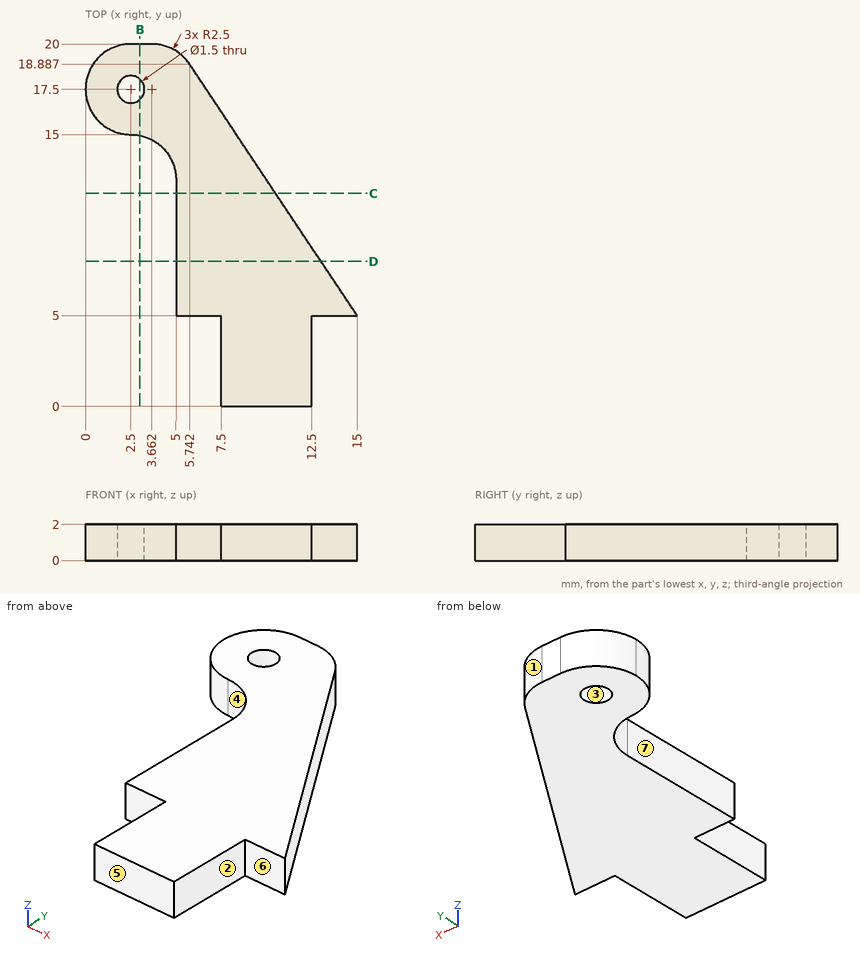
Part print with two shaded views. Sizes in mm from the minimum x, y, z corner. A direction names the side the tool comes from. Coordinates: 2 decimals unless noted, no trailing zeros. Write each loop counter-clockwise with the first axis right and the second up, starting at its lowest first coordinate (ties: lowest second). Pieces come first, ordered by that corner, then holes. Notation, with made-up numbers: (-16.5, 0.5) -> (0.5, 0.5) arc R31 ccw to (0.5, 25.5) -> close; hole circle Ø4 at (8, 9.5). An arc over 180 degrees is marked (long way). Return JSON: item names as keys, results as strings. Group by question number.
Q1. Drill centre lines: line 1 (Y direction, x = 2.5, z = 1.35); line 2 (X direction, y = 1.75, z = 1.2); line 3 (X direction, y = 17.75, z = 1.2). Where is each one in solid material? Low to high.
Q2. Cut at D-D, the plane y = 8. Give the cut face in (x, z), then the cut area to 3 significant figures.
Q3. Cut at C-C, the plane y = 11.75. Give the cut face in (x, z), then the cut area to 3 significant figures.
Q4. Which spindle directions (+Z, -Z, +X, -X, +Y, -Y) get a long thin tool onto all of the face, cutting with end or side? Do the marked faces 5, 6 and 7. Say none if no direction does.
Q5. Cut at B-B, the plane x = 3. Give the cut face in (y, z).
Q6. Pull direction Y, two halves, no side cores. Call the marked faces 1, 2, 3 and 4: released by +Y, released by -Y, zero draft, split by the parting line, or undercut.
Q7. Flat gauge pins, fed straight in: pin 1 (1 mm diameter, centred on x = 14, z = 0.5, fed in from -Y); pin 2 (0.6 mm diameter, centred on y = 3, z = 1, fed in from +X); pin 3 (1 mm diameter, centred on y = 2.5, z = 1.5, fed in from -X). Where does each tip first touch, or does it go through?
Returned:
{
 "1": {"line 1": "y = 15 to 16.75, 18.25 to 20", "line 2": "x = 7.5 to 12.5", "line 3": "x = 0.01 to 1.79, 3.21 to 6.5"},
 "2": {"outline": "(5, 0) -> (13, 0) -> (13, 2) -> (5, 2) -> close", "area": "16.0 mm2"},
 "3": {"outline": "(5, 0) -> (10.5, 0) -> (10.5, 2) -> (5, 2) -> close", "area": "11.0 mm2"},
 "4": {"face 5": "+Z, -Z, +X, -X, -Y", "face 6": "+Z, -Z, +X, -Y", "face 7": "+Z, -Z, -X, -Y"},
 "5": {"outline": "(14.95, 0) -> (16.94, 0) -> (16.94, 2) -> (14.95, 2) -> close; (18.06, 0) -> (20, 0) -> (20, 2) -> (18.06, 2) -> close"},
 "6": {"face 1": "released by +Y", "face 2": "zero draft", "face 3": "undercut", "face 4": "released by -Y"},
 "7": {"pin 1": "stops at y = 5", "pin 2": "stops at x = 12.5", "pin 3": "stops at x = 7.5"}
}
